```python
from build123d import *

# Parameters (mm, degrees)
F1_DEPTH = 11
F2_T     = -3
F3_R     = 2
F4_R     = 2


with BuildPart() as f1:
    # F0 (on Top) → F1 (new body)
    with BuildSketch(Plane.XY):
        with BuildLine():
            Line((21.98791, -21.934712), (21.98791, 63.065288))
            ThreePointArc((21.98791, 63.065288), (3.98791, 81.065288), (-14.01209, 63.065288))
            Line((-14.01209, 63.065288), (-14.01209, -21.934712))
            Line((-14.01209, -21.934712), (21.98791, -21.934712))
        make_face()
    extrude(amount=F1_DEPTH)

    # F2
    f2_openings = [f1.faces().sort_by_distance(p)[0] for p in [
        (3.98791, -21.934712, 5.5),
    ]]
    offset(amount=F2_T, openings=f2_openings)

    # F3
    f3_edges = [f1.edges().sort_by_distance(p)[0] for p in [
        (-14.01209, 20.565288, 11),
        (3.98791, 81.065288, 11),
        (21.98791, 20.565288, 11),
    ]]
    fillet(f3_edges, radius=F3_R)

    # F4
    f4_edges = [f1.edges().sort_by_distance(p)[0] for p in [
        (-14.01209, 20.565288, 0),
        (21.98791, 20.565288, 0),
        (3.98791, 81.065288, 0),
    ]]
    fillet(f4_edges, radius=F4_R)


solid = f1.part
```
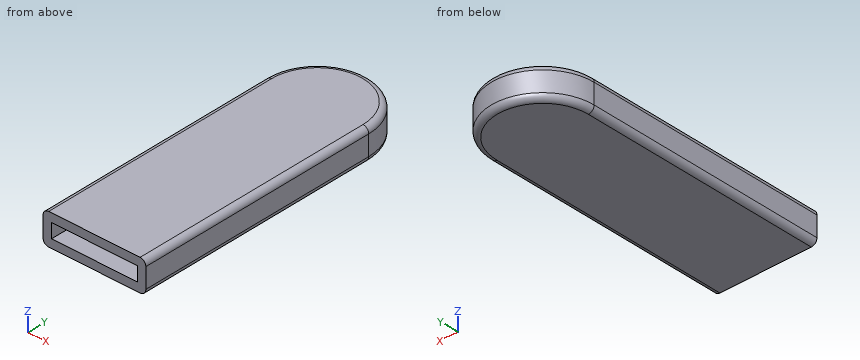
Geometry: final body of the model. Coordinates: model frame, mm. Coordinates: 2 decimals unless noted, no trailing zeros. Order: outer loops, then holes, each group sorted by start corner. A loop starts at its lowest first (then second) coordinate and runs counter-clockwise, first axis right, second up. Notation, with made-up numbers: (7.25, 28.25) - (25.25, 28.25) arc R16 ccw to (25.25, 45.25) - close; hole circle Ø2 at (14.5, 34). An arc over 180 degrees is marked (long way). Write each question's results on one line, items separated by ' | '.
1) Section C-C, the plane z = 1. Return loops of the section in (x, y).
Results list:
outline: (-13.74, -21.93) - (21.72, -21.93) - (21.72, 63.07) arc R17.73 ccw to (-13.74, 63.07) - close
2) Section B-B, the plane z = 5.5. Return loops of the section in (x, y), plus the area to 3 significant figures.
Results list:
outline: (-14.01, -21.93) - (-11.01, -21.93) - (-11.01, 63.07) arc R15 cw to (18.99, 63.07) - (18.99, -21.93) - (21.99, -21.93) - (21.99, 63.07) arc R18 ccw to (-14.01, 63.07) - close | area: 666 mm^2
3) Line query: line 1 (Z direction, x = -9, y = 11); line 2 (X direction, y = -17, z = 6); line 3 (X direction, y = 10.5, z = 0.75). Output: solid intervals per line, ascending. Write a range as from..to.
Results list:
line 1: 0..3, 8..11 | line 2: -14.01..-11.01, 18.99..21.99 | line 3: -13.57..21.55
4) Pin query (flat end, axial travel): pin 1 (1.5 mm diameter, centred on x = 3.5, z = 6.5, fed in from -Y); pin 2 (5 mm diameter, centred on x = -5.5, z = 10, fed in from +Y); pin 3 (1 mm diameter, centred on x = -2, z = 4, fed in from -Y). Return the tip coordinate at first contact, or that it passes through.
Results list:
pin 1: y = 78.01 | pin 2: y = 79.59 | pin 3: y = 76.59
5) Section A-A, the plane y = 61. Return loops of the section in (x, z), plus the area to 3 significant figures.
Results list:
outline: (-14.01, 2) arc R2 ccw to (-12.01, 0) - (19.99, 0) arc R2 ccw to (21.99, 2) - (21.99, 9) arc R2 ccw to (19.99, 11) - (-12.01, 11) arc R2 ccw to (-14.01, 9) - close; hole (-11.01, 3) - (18.99, 3) - (18.99, 8) - (-11.01, 8) - close | area: 243 mm^2
